Could you check a few things on this model? Use its own coordinates, in mm. A direction names the side the tool comes from. Round coordinates to 2 decimals unless told otherwise and drop trailing zeros. Order: outer loops, then holes, each group sorted by start corner. A loop starts at its lowest first (then second) coordinate and runs counter-clockwise, first axis right, second up. Notation, with made-up numbers: (38, 1) -> (87, 1) arc R16 ccw to (87, 18) -> close; hole circle Ø2 at (-5.75, -15). An arc over 180 degrees is marked (long way). One line per question, with ' | ' between items.
```python
from build123d import *

# Parameters (mm, degrees)
SKETCH_1_W          = 117
SKETCH_1_H          = 60
EXTRUDE_1_DEPTH     = 17
SKETCH_2_W          = 102
SKETCH_2_H          = 45
CUT_EXTRUDE_1_DEPTH = 15
SKETCH_4_R          = 1.7
CUT_EXTRUDE_2_DEPTH = 18
SKETCH_5_W          = 7.5
SKETCH_5_H          = 7.5
CUT_EXTRUDE_3_DEPTH = 6
FILLET_2_R          = 1


with BuildPart() as part:
    # ｽｹｯﾁ1 → ﾎﾞｽ - 押し出し1 (new body)
    with BuildSketch(Plane.XY):
        Rectangle(SKETCH_1_W, SKETCH_1_H)
    extrude(amount=EXTRUDE_1_DEPTH)

    # ｽｹｯﾁ2 → ｶｯﾄ - 押し出し1 (cut)
    with BuildSketch(Plane.XY.offset(17)):
        Rectangle(SKETCH_2_W, SKETCH_2_H)
    extrude(amount=-CUT_EXTRUDE_1_DEPTH, mode=Mode.SUBTRACT)

    # ｽｹｯﾁ4 → ｶｯﾄ - 押し出し2 (cut, through all)
    with BuildSketch(Plane(origin=(0, 0, 0), x_dir=(-1, 0, 0), z_dir=(0, 0, -1))):
        with Locations((15, 26.25)):
            Circle(SKETCH_4_R)
        with Locations((15, -26.25)):
            Circle(SKETCH_4_R)
        with Locations((-48.5, -26.25)):
            Circle(SKETCH_4_R)
        with Locations((-48.5, 26.25)):
            Circle(SKETCH_4_R)
    extrude(amount=-CUT_EXTRUDE_2_DEPTH, mode=Mode.SUBTRACT)

    # ｽｹｯﾁ5 → ｶｯﾄ - 押し出し3 (cut)
    with BuildSketch(Plane(origin=(0, 0, 0), x_dir=(-1, 0, 0), z_dir=(0, 0, -1))):
        with Locations((-48.5, -26.25)):
            Rectangle(SKETCH_5_W, SKETCH_5_H)
        with Locations((-48.5, 26.25)):
            Rectangle(SKETCH_5_W, SKETCH_5_H)
        with Locations((15, 26.25)):
            Rectangle(SKETCH_5_W, SKETCH_5_H)
        with Locations((15, -26.25)):
            Rectangle(SKETCH_5_W, SKETCH_5_H)
    extrude(amount=-CUT_EXTRUDE_3_DEPTH, mode=Mode.SUBTRACT)

    # ﾌｨﾚｯﾄ2
    fillet_2_edges = [part.edges().sort_by_distance(p)[0] for p in [
        (55.375, 30, 0),
        (58.5, 0, 0),
        (16.75, 30, 0),
        (-38.625, 30, 0),
        (16.75, -30, 0),
        (55.375, -30, 0),
        (-38.625, -30, 0),
        (-58.5, 0, 0),
        (-18.75, -26.25, 0),
        (-15, -22.5, 0),
        (-11.25, -26.25, 0),
        (-18.75, 26.25, 0),
        (-11.25, 26.25, 0),
        (-15, 22.5, 0),
        (44.75, 26.25, 0),
        (52.25, 26.25, 0),
        (48.5, 22.5, 0),
        (44.75, -26.25, 0),
        (48.5, -22.5, 0),
        (52.25, -26.25, 0),
    ]]
    fillet(fillet_2_edges, radius=FILLET_2_R)


solid = part.part
```
1. On a 3-axis mill with a long thin cutter (end or side, diameter ignored), from which of +Z, -Z, +X, -X, +Y, -Y can I reach the whole of each face in a straight line? I mean faces 5 (the face through (-15.914, 27.683, 11.423)), 6 (the face through (51, 0, 10)), 7 (the face through (44.75, 26, 3)), 8 (the face through (-1, 0, 0)), 9 (the face through (49.4, -24.5, 6)). Say none if no direction works.
From the geometry:
face 5: +Z, -Z | face 6: +Z | face 7: -Z, +Y | face 8: -Z, +X, -X, +Y, -Y | face 9: -Z, -Y
2. I want a section at C-C on y = -26.25. List the corners of the cut face in (x, z) for me, and give its area (3 significant figures).
From the geometry:
outline: (-58.5, 1) arc R1 ccw to (-57.5, 0) -> (-19.75, 0) arc R1 ccw to (-18.75, 1) -> (-18.75, 6) -> (-16.7, 6) -> (-16.7, 17) -> (-58.5, 17) -> close; (-13.3, 6) -> (-11.25, 6) -> (-11.25, 1) arc R1 ccw to (-10.25, 0) -> (43.75, 0) arc R1 ccw to (44.75, 1) -> (44.75, 6) -> (46.8, 6) -> (46.8, 17) -> (-13.3, 17) -> close; (50.2, 6) -> (52.25, 6) -> (52.25, 1) arc R1 ccw to (53.25, 0) -> (57.5, 0) arc R1 ccw to (58.5, 1) -> (58.5, 17) -> (50.2, 17) -> close | area: 1,820 mm²
3. I want a section at A-A on x = 48.5. List the corners of the cut face in (y, z) for me, and give its area (3 significant figures).
From the geometry:
outline: (-30, 6) -> (-27.95, 6) -> (-27.95, 17) -> (-30, 17) -> close; (-24.55, 6) -> (-22.5, 6) -> (-22.5, 17) -> (-24.55, 17) -> close; (-22.5, 1) arc R1 ccw to (-21.5, 0) -> (21.5, 0) arc R1 ccw to (22.5, 1) -> (22.5, 2) -> (-22.5, 2) -> close; (22.5, 6) -> (24.55, 6) -> (24.55, 17) -> (22.5, 17) -> close; (27.95, 6) -> (30, 6) -> (30, 17) -> (27.95, 17) -> close | area: 180 mm²
4. I want a section at D-D on y = -3. List the corners of the cut face in (x, z) for me, and give its area (3 significant figures).
From the geometry:
outline: (-58.5, 1) arc R1 ccw to (-57.5, 0) -> (57.5, 0) arc R1 ccw to (58.5, 1) -> (58.5, 17) -> (51, 17) -> (51, 2) -> (-51, 2) -> (-51, 17) -> (-58.5, 17) -> close | area: 459 mm²
5. I want a section at B-B on z = 7.75. List the corners of the cut face in (x, y) for me, and give its area (3 significant figures).
From the geometry:
outline: (-58.5, -30) -> (58.5, -30) -> (58.5, 30) -> (-58.5, 30) -> close; hole (-51, -22.5) -> (51, -22.5) -> (51, 22.5) -> (-51, 22.5) -> close; hole circle Ø3.4 at (-15, -26.25); hole circle Ø3.4 at (-15, 26.25); hole circle Ø3.4 at (48.5, -26.25); hole circle Ø3.4 at (48.5, 26.25) | area: 2,390 mm²
6. If we mould it in two halves opening along Y, with no side actions, what happens to faces 1 (the face through (-1, -30, 9)), 2 (the face through (49.75, 27.4, 11.42)), 3 (the face through (-18.75, -26, 3)), 4 (the face through (-1, -22.5, 10))? For each: pulls with the +Y half, pulls with the -Y half, needs draft (parallel to the pull), parting line crosses it, or undercut.
From the geometry:
face 1: pulls with the -Y half | face 2: undercut | face 3: needs draft | face 4: undercut
7. I'm going to push flat-ended pins straight in: pin 1 (4 mm diameter, centred on x = 50, y = -25.5, fed in from -Z); pin 2 (0.8 mm diameter, centred on x = -14, z = 1.5, fed in from -Y); pin 3 (1.5 mm diameter, centred on x = -11, y = -21.5, fed in from +Z). Where does each tip first touch, or does it pass through?
From the geometry:
pin 1: stops at z = 6 | pin 2: stops at y = -22.5 | pin 3: stops at z = 2
8. I need wall thicknesses on probe 1 along X at (y, z) = (-25, 2); probe 2 along Y at (x, z) = (48.5, 11.25); probe 3 along Y at (x, z) = (-45.5, 8). Which ranges of each line are inside material? Lowest first, please.
From the geometry:
probe 1: x = -58.5 to -18.75, -11.25 to 44.75, 52.25 to 58.5 | probe 2: y = -30 to -27.95, -24.55 to -22.5, 22.5 to 24.55, 27.95 to 30 | probe 3: y = -30 to -22.5, 22.5 to 30
